The drawing under review shows one solid part. Ordinate dimensions are in mm from its lowest x, y, z. A direction names the side the tool comes from. Coordinates: 2 decimals unless noted, no trailing zeros. Write each loop counter-clockwise with the first axis right and the second up, starting at its lowest first coordinate (ties: lowest second). Pieces come first, ordered by that corner, then holes.
Q1. Add section A-A, the plane x = 40. Give the boundary of the cut face in (y, z), plus the area to 3 significant figures.
Q2. Add section B-B, the plane z = 17. Give the boundary of the cut face in (x, y).
Q3. Clearance check with flat-ended pins moving along their axes: pin 1 Ø1.5 at (y, z) = (66, 11.5) entering from -X; pin 2 Ø10 at (y, z) = (20.5, 6) entering from +X; pin 3 Ø1 at (y, z) = (11.5, 6) entering from +X. State where each tip first meets the part, or that it passes through.
Q4. Machinability: for the marked faces 1, 2 and 3, which of the approach directions +Z, -Z, +X, -X, +Y, -Y give a long, thin tool a straight path to every point of the face, cutting with its end or side? Answer none if there is none.
Q5. To check wall thickness, follow probe 1 along Z at (x, y) = (13.5, 68.5); probe 2 along Y at (x, z) = (15, 6.25); probe 3 along Y at (x, z) = (46, 19). State the ranges of each line that lie inside material, in increasing order.
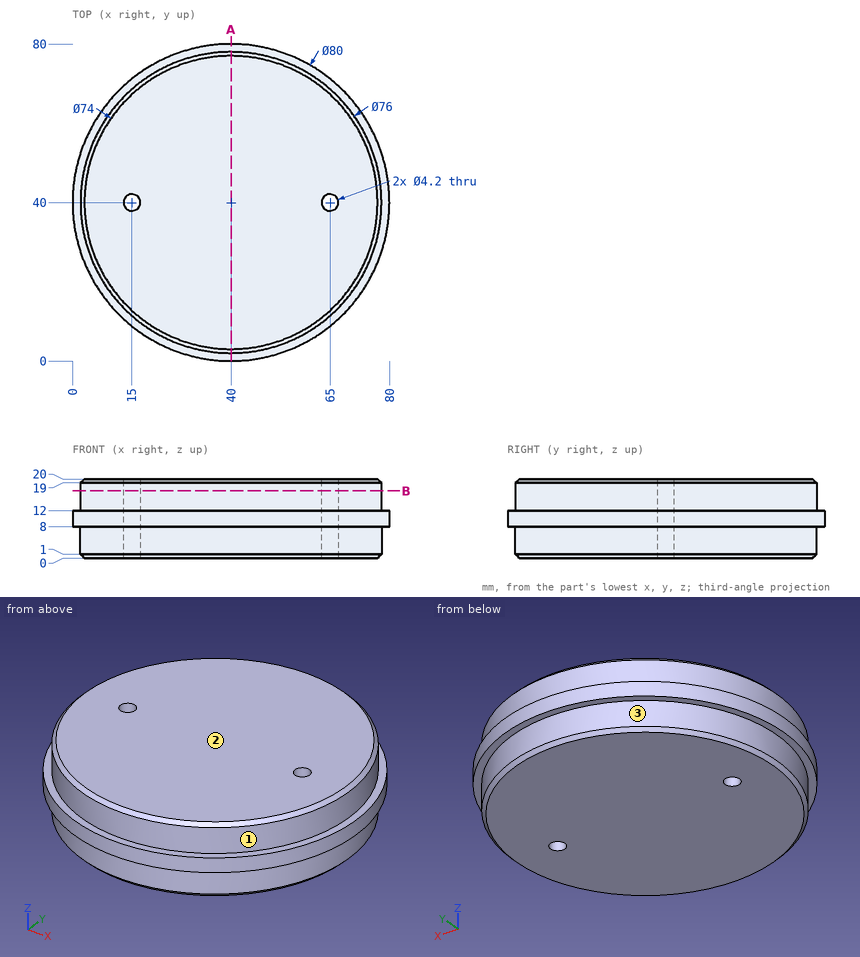
Here are the results:
1. outline: (0, 8) - (2, 8) - (2, 1) - (3, 0) - (77, 0) - (78, 1) - (78, 8) - (80, 8) - (80, 12) - (78, 12) - (78, 19) - (77, 20) - (3, 20) - (2, 19) - (2, 12) - (0, 12) - close
1. area: 1,530 mm2
2. outline: circle Ø76 at (40, 40); hole circle Ø4.2 at (15, 40); hole circle Ø4.2 at (65, 40)
3. pin 1: stops at x = 8.98
3. pin 2: stops at x = 77.11
3. pin 3: stops at x = 65.69
4. face 1: +Z
4. face 2: +Z, +X, -X, +Y, -Y
4. face 3: -Z
5. probe 1: z = 8 to 12
5. probe 2: y = 11.38 to 37.9, 42.1 to 68.62
5. probe 3: y = 2.48 to 77.52
